Part model, mm, in its own coordinate system. Face numbers are marked on the shaded views. Round coordinates to 2 decimals unless told otherwise and drop trailing zeros. Write each loop counter-clockwise with the first axis right and the second up, starting at its lowest first coordinate (ties: lowest second). Pieces come first, ordered by that corner, then holes. Notation, with made-up numbers: M 26.25,-36.75 L 74.25,-36.75 A20 ccw 74.25,-26.75 Z; hole C 6,-37 d11. An arc over 180 degrees is marked long. Use one line per item in the form item = value. Start each with the question number.
Item 1: Flat gauge pins, fed straight in: pin 1 Ø1 at (x, z) = (-8.5, 12.5) entering from -Y; pin 2 Ø3.5 at (x, z) = (0, 17) entering from +Y; pin 3 Ø2 at (y, z) = (-13, 5.5) entering from +X. Where does each tip first touch, or does it go through?
Item 2: Cut at D-D, the plane y = -18. Give the cut face in (x, z), then the cut area to 3 significant figures.
Item 3: Mould opens along Z. For the marked faces 1, 2 and 3 say: +Z half, -Z half, draft (parallel to the pull), parting line (faces both ways), or undercut.
Item 4: Cut at C-C, the plane z = 17. Give the cut face in (x, y).
Item 5: Cut at B-B, the plane y = 9. Give the cut face in (x, z).
Item 6: Cut at A-A, the plane x = 0. Give the cut face in (y, z), then the cut area to 3 significant figures.
Item 7: Probe L1, parallel to Z at x = -0.25, y = -5; L2, parallel to Z at x = -2, y = 3.5; L3, parallel to Z at x = 8.25, y = 9. List the from-to ranges inside material, lowest first.
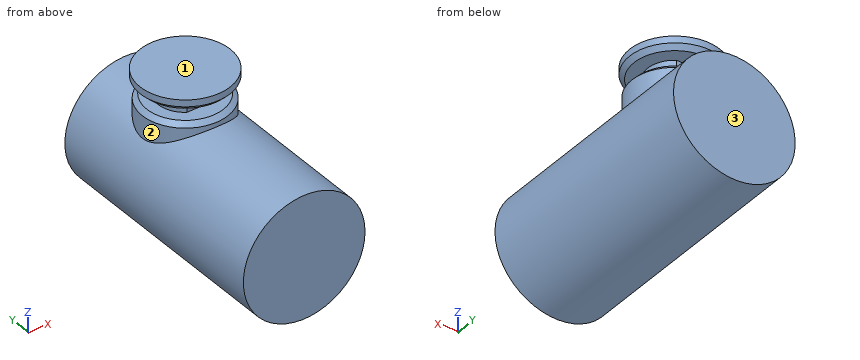
from build123d import *

# Parameters (mm, degrees)
F0_R     = 13.5
F1_DEPTH = 27
F3_R     = 9.5
F5_SIZE  = 1
F7_DEPTH = 3
F8_R     = 10
F9_DEPTH = 2.5
F10_SIZE = 1


with BuildPart() as f1:
    # F0 (on Front) → F1 (new body, symmetric)
    with BuildSketch(Plane.XZ):
        Circle(F0_R)
    extrude(amount=F1_DEPTH, both=True)

    # F3 (on offset) → F4 (join, up to the next surface of F1)
    with BuildSketch(Plane.XY.offset(15.5)):
        with Locations((0, 9)):
            Circle(F3_R)
    extrude(until=Until.NEXT, dir=(0, 0, -1))

    # F5
    f5_edges = [f1.edges().sort_by_distance(p)[0] for p in [
        (-9.5, 9, 15.5),
    ]]
    chamfer(f5_edges, length=F5_SIZE)

    # F6 (on face) → F7 (join)
    with BuildSketch(Plane.XY.offset(15.5)):
        with BuildLine():
            Line((3.3166247904, 14), (-3.3166247904, 14))
            ThreePointArc((-3.3166247904, 14), (-6, 9), (-3.3166247904, 4))
            Line((-3.3166247904, 4), (3.3166247904, 4))
            ThreePointArc((3.3166247904, 4), (6, 9), (3.3166247904, 14))
        make_face()
    extrude(amount=F7_DEPTH)

    # F8 (on face) → F9 (join)
    with BuildSketch(Plane.XY.offset(18.5)):
        with Locations((0, 9)):
            Circle(F8_R)
    extrude(amount=F9_DEPTH)

    # F10
    f10_edges = [f1.edges().sort_by_distance(p)[0] for p in [
        (-10, 9, 18.5),
    ]]
    chamfer(f10_edges, length=F10_SIZE)


solid = f1.part
Model answer:
q1.pin_1 = 3.88
q1.pin_2 = 18.25
q1.pin_3 = 12.73
q2.outline = C 0,0 d27
q2.area = 573 mm²
q3.face_1 = +Z half
q3.face_2 = undercut
q3.face_3 = draft
q4.outline = M -3.32,4 L 3.32,4 A6 ccw 3.32,14 L -3.32,14 A6 ccw Z
q5.outline = M -10,19.5 L -9,18.5 L -6,18.5 L -6,15.5 L -8.5,15.5 L -9.5,14.5 L -9.5,9.59 A13.5 ccw long 9.5,9.59 L 9.5,14.5 L 8.5,15.5 L 6,15.5 L 6,18.5 L 9,18.5 L 10,19.5 L 10,21 L -10,21 Z
q6.outline = M -27,-13.5 L 27,-13.5 L 27,13.5 L 18.5,13.5 L 18.5,14.5 L 17.5,15.5 L 14,15.5 L 14,18.5 L 18,18.5 L 19,19.5 L 19,21 L -1,21 L -1,19.5 L 0,18.5 L 4,18.5 L 4,15.5 L 0.5,15.5 L -0.5,14.5 L -0.5,13.5 L -27,13.5 Z
q6.area = 1,570 mm²
q7.L1 = -13.5 to 13.5
q7.L2 = -13.35 to 15.5, 18.5 to 21
q7.L3 = -10.69 to 15.5, 18.5 to 21
